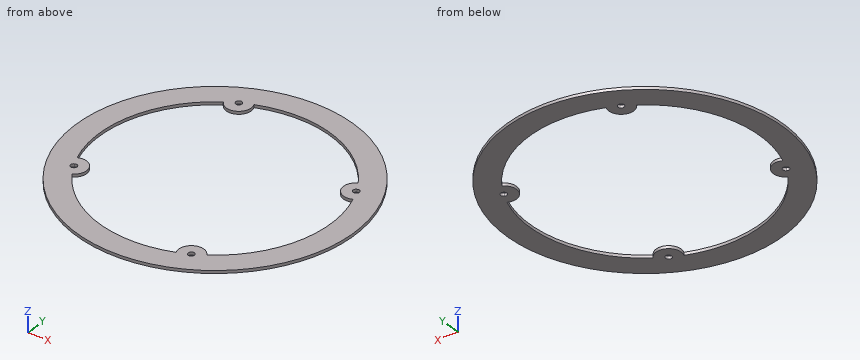
from build123d import *

# Parameters (mm, degrees)
SKETCH1_R           = 76.2
SKETCH1_R_2         = 63.5
BOSS_EXTRUDE1_DEPTH = 1.5875
SKETCH2_R           = 1.651
BOSS_EXTRUDE2_DEPTH = 1.5875
SKETCH4_R           = 1.651
CUT_EXTRUDE2_DEPTH  = 1.5875
CIRPATTERN2_COUNT   = 4
CIRPATTERN3_COUNT   = 4


with BuildPart() as part:
    # Sketch1 → Boss-Extrude1 (new body)
    with BuildSketch(Plane.XY):
        Circle(SKETCH1_R)
        Circle(SKETCH1_R_2, mode=Mode.SUBTRACT)
    extrude(amount=BOSS_EXTRUDE1_DEPTH)

    # Sketch2 → Boss-Extrude2 (add)
    with BuildSketch(Plane.XY.offset(1.5875)):
        with BuildLine():
            Line((-36.496083221, 54.681087122), (-25.299953382, 61.158320597))
            ThreePointArc((-25.299953382, 61.158320597), (-26.271105519, 49.921919547), (-36.496083221, 54.681087122))
        make_face()
        with Locations((-29.718, 55.88)):
            Circle(SKETCH2_R, mode=Mode.SUBTRACT)
    boss_extrude2 = extrude(amount=-BOSS_EXTRUDE2_DEPTH)

    # Sketch4 → Cut-Extrude2 (cut)
    with BuildSketch(Plane.XY.offset(1.5875)):
        with Locations((-29.81619736, 56.064644608)):
            Circle(SKETCH4_R)
    cut_extrude2 = extrude(amount=-CUT_EXTRUDE2_DEPTH, mode=Mode.SUBTRACT)

    # CirPattern2: Boss-Extrude2 ×4 about axis
    cirpattern2_axis = Axis((0, 0, 0), (0, 0, 1))
    for i in range(1, CIRPATTERN2_COUNT):
        add(boss_extrude2.rotate(cirpattern2_axis, i * 360 / CIRPATTERN2_COUNT))

    # CirPattern3: Cut-Extrude2 ×4 about axis
    cirpattern3_axis = Axis((0, 0, 0), (0, 0, 1))
    for i in range(1, CIRPATTERN3_COUNT):
        add(cut_extrude2.rotate(cirpattern3_axis, i * 360 / CIRPATTERN3_COUNT), mode=Mode.SUBTRACT)


solid = part.part
Work out the finished part from the listing and answer in its coordinate system (mm). Give positions to 0.01 mm unless a question says otherwise; leave off trailing zeros. Loops run counter-clockwise (first coordinate to the right, second up) from the corner with the lowest first, then second, coordinate; pieces in that order, holes last. Notation, with made-up numbers: (3.5, 76.5) - (29.5, 76.5) arc R26 cw to (29.5, 100.5) - close; hole circle Ø5 at (62.25, 89). An arc over 180 degrees is marked (long way). Answer in a Markdown table with one row per item. Add a question column.
Q1. The part is cut by section C-C (z = 0.4). Determine the outline of the cut face in (x, y), and give its area (3 significant figures).
Q2. The part is cut by section A-A (x = 0). Determine the outline of the cut face in (y, z).
Q3. Consider line 1 along X through (y, z) = (-57, 0.2); line 2 along Y through (x, z) = (-0.5, 1.3); line 3 along Y through (x, z) = (-55.5, 0.95). Determine where each line is inside the solid, lowest interval first.
Solution:
| question | item | result |
|---|---|---|
| 1 | outline | circle Ø152.4 at (0, 0); hole (-58.97, -23.57) arc R6.88 cw to (-52.5, -35.72) arc R63.5 ccw to (23.57, -58.97) arc R6.88 cw to (35.72, -52.5) arc R63.5 ccw to (58.97, 23.57) arc R6.88 cw to (52.5, 35.72) arc R63.5 ccw to (-23.57, 58.97) arc R6.88 cw to (-35.72, 52.5) arc R63.5 ccw to start; hole (-56.75, -28.31) arc R1.65 ccw (long way) to (-55.2, -31.22) arc R1.65 ccw (long way) to start; hole (-31.22, 55.2) arc R1.65 ccw (long way) to (-28.31, 56.75) arc R1.65 ccw (long way) to start; hole (28.31, -56.75) arc R1.65 ccw (long way) to (31.22, -55.2) arc R1.65 ccw (long way) to start; hole (55.2, 31.22) arc R1.65 ccw (long way) to (56.75, 28.31) arc R1.65 ccw (long way) to start |
| 1 | area | 5,840 mm² |
| 2 | outline | (-76.2, 0) - (-63.5, 0) - (-63.5, 1.59) - (-76.2, 1.59) - close; (63.5, 0) - (76.2, 0) - (76.2, 1.59) - (63.5, 1.59) - close |
| 3 | line 1 | x = -50.57 to -27.99, 22.93 to 28.46, 31.18 to 50.57 |
| 3 | line 2 | y = -76.2 to -63.5, 63.5 to 76.2 |
| 3 | line 3 | y = -52.21 to -31.37, -28.11 to -22.85, 30.85 to 52.21 |
